from build123d import *

# Parameters (mm, degrees)
EXTRUDE_1_DEPTH     = 10
SKETCH_2_R          = 1.65
CUT_EXTRUDE_1_DEPTH = 45.653083029
SKETCH_4_R          = 1.65
CUT_EXTRUDE_3_DEPTH = 10
SKETCH_5_R          = 3.05
CUT_EXTRUDE_4_DEPTH = 10
FILLET_2_R          = 2


with BuildPart() as part:
    # ｽｹｯﾁ1 → ﾎﾞｽ - 押し出し1 (new body)
    with BuildSketch(Plane(origin=(0, 0, 0), x_dir=(1, 0, 0), z_dir=(0, 1, 0))):
        Polygon((-25, 5), (8, 5), (31.233495706, 28.233495706), (24.162427894, 35.304563517), (3.857864376, 15), (-25, 15), align=None)
    extrude(amount=EXTRUDE_1_DEPTH)

    # ｽｹｯﾁ2 → ｶｯﾄ - 押し出し1 (cut, through all)
    with BuildSketch(Plane.XY.offset(-5)):
        with Locations((-20, 5)):
            Circle(SKETCH_2_R)
        with Locations((0, 5)):
            Circle(SKETCH_2_R)
    extrude(amount=-CUT_EXTRUDE_1_DEPTH, mode=Mode.SUBTRACT)

    # ｽｹｯﾁ4 → ｶｯﾄ - 押し出し3 (cut)
    with BuildSketch(Plane(origin=(1.5, 0, 1.5), x_dir=(0.7071067811865472, 0, -0.7071067811865479), z_dir=(0.7071067811865479, 0, 0.7071067811865472))):
        with Locations((37.049512883, 5)):
            Circle(SKETCH_4_R)
        with Locations((17.049512883, 5)):
            Circle(SKETCH_4_R)
    extrude(amount=-CUT_EXTRUDE_3_DEPTH, mode=Mode.SUBTRACT)

    # ｽｹｯﾁ5 → ｶｯﾄ - 押し出し4 (cut)
    with BuildSketch(Plane(origin=(0, 10, 0), x_dir=(1, 0, 0), z_dir=(0, 1, 0))):
        with Locations(Location((5.928932188, 10, 0), (0, 0, 270))):
            Circle(SKETCH_5_R)
        with BuildLine():
            Line((-14.5, 13.05), (-5.5, 13.05))
            ThreePointArc((-5.5, 13.05), (-2.45, 10), (-5.5, 6.95))
            Line((-5.5, 6.95), (-14.5, 6.95))
            ThreePointArc((-14.5, 6.95), (-17.55, 10), (-14.5, 13.05))
        make_face()
        with BuildLine():
            Line((22.43001628, 22.187732726), (16.066055249, 15.823771696))
            ThreePointArc((16.066055249, 15.823771696), (11.752703884, 15.823771696), (11.752703884, 20.137123061))
            Line((11.752703884, 20.137123061), (18.116664914, 26.501084092))
            ThreePointArc((18.116664914, 26.501084092), (22.43001628, 26.501084092), (22.43001628, 22.187732726))
        make_face()
    extrude(amount=-CUT_EXTRUDE_4_DEPTH, mode=Mode.SUBTRACT)

    # ﾌｨﾚｯﾄ2
    fillet_2_edges = [part.edges().sort_by_distance(p)[0] for p in [
        (-25, 5, -15),
        (3.857864376, 5, -15),
        (24.162427894, 5, -35.304563517),
        (31.233495706, 5, -28.233495706),
        (8, 5, -5),
        (-25, 5, -5),
    ]]
    fillet(fillet_2_edges, radius=FILLET_2_R)


solid = part.part
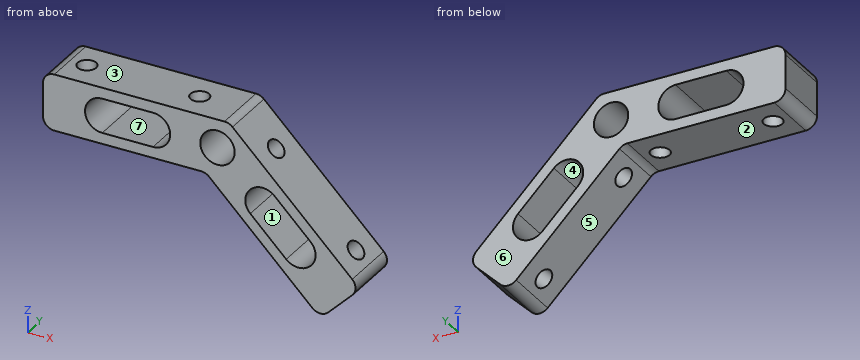
The listing builds one solid part. Answer for the finished solid, in the listing's coordinates (mm). Face numbers are marked on the shaded views. A direction names the side the tool comes from. Coordinates: 2 decimals unless noted, no trailing zeros. Loops run counter-clockwise (first coordinate to the right, second up) from the corner with the lowest first, then second, coordinate; pieces in that order, holes last. Notation, with made-up numbers: (31, 8) -> (79, 8) arc R38 ccw to (79, 46) -> close; hole circle Ø8 at (12.5, 56.5). An arc over 180 degrees is marked (long way). Write item = value, one per line. Start each with the question number.
1) A cutting plane is placed at B-B (x = -20). Give the vertices of the cut face in (y, z), then the cut area to 3 significant figures.
2) Straight lines are drawn through the part: line 1 (X direction, y = 3, z = -10); line 2 (Z direction, x = -10, y = 6); line 3 (Y direction, x = 0, z = -7.5). For each, find the intervals that lie inside material, in ascending order. Write a range as from..to.
3) A cutting plane is placed at D-D (y = 7.25). Give the vertices of the cut face in (x, z).
4) A cutting plane is placed at A-A (x = -8). Give the vertices of the cut face in (y, z).
5) A tool of negligible diameter and unlimited length cuts with its end or side. For the marked faces 1, 2 and 3, from which of +Z, -Z, +X, -X, +Y, -Y can it reach the whole face along a straight path? Write none if from no direction.
6) A cutting plane is placed at C-C (z = -10). Count the separate pieces of the cut face and the enclosed holes in it, then the cut area to 3 significant figures.
7) The mould has two halves that part along Z. Classify the marked faces 4, 5, 6 and 7: released by +Z, released by -Z, zero draft, split by the parting line, or undercut.
8) Given pin 1 Ø3 at (x, y) = (-13.5, 3.5) entering from -Z; pin 2 Ø1 at (y, z) = (3, -25) entering from -X; pin 3 Ø2 at (x, z) = (-17, -12.5) entering from -Y, each flat-ended and moving along its own axis, determine where each tip first touches the part or whether it passes through.
Responses:
q1.outline = (0, -15) -> (3.35, -15) -> (3.35, -5) -> (0, -5) -> close; (6.65, -15) -> (10, -15) -> (10, -5) -> (6.65, -5) -> close
q1.area = 67.0 mm²
q2.line_1 = -25..-17.55, -2.45..2.88, 8.98..13
q2.line_2 = -15..-13.05, -6.95..-5
q2.line_3 = 0..3.35, 6.65..10
q3.outline = (-25, -13) arc R2 ccw to (-23, -15) -> (3.03, -15) arc R2 cw to (4.44, -15.59) -> (22.75, -33.89) arc R2 ccw to (25.58, -33.89) -> (29.82, -29.65) arc R2 ccw to (29.82, -26.82) -> (8.59, -5.59) arc R2 ccw to (7.17, -5) -> (-23, -5) arc R2 ccw to (-25, -7) -> close; hole (-14.5, -13.05) -> (-5.5, -13.05) arc R3.05 ccw to (-5.5, -6.95) -> (-14.5, -6.95) arc R3.05 ccw to start; hole circle Ø6.1 at (5.93, -10); hole (11.75, -20.14) -> (18.12, -26.5) arc R3.05 ccw to (22.43, -22.19) -> (16.07, -15.82) arc R3.05 ccw to start
q4.outline = (0, -15) -> (10, -15) -> (10, -13.05) -> (0, -13.05) -> close; (0, -6.95) -> (10, -6.95) -> (10, -5) -> (0, -5) -> close
q5.face_1 = +Y, -Y
q5.face_2 = -Z, -X, +Y, -Y
q5.face_3 = +Z, +X, -X, +Y, -Y
q6.separate_pieces = 3
q6.enclosed_holes = 2
q6.area = 148 mm²
q7.face_4 = undercut
q7.face_5 = released by -Z
q7.face_6 = zero draft
q7.face_7 = undercut
q8.pin_1 = -15
q8.pin_2 = 13.36
q8.pin_3 = 0
